Part model, mm, in its own coordinate system. Face numbers are marked on the shaded views. A direction names the side the tool comes from. Give positions to 0.01 mm unless a question says otherwise; leave off trailing zeros. Order: outer loops, then holes, each group sorted by start corner. A loop starts at its lowest first (then second) coordinate and runs counter-clockwise, first axis right, second up. Notation, with made-up numbers: (41, -6.5) -> (67, -6.5) arc R28 ccw to (67, 30.5) -> close; hole circle Ø6 at (23.5, -8.75). An arc over 180 degrees is marked (long way). Write item = value, one per line. Start each with the question number.
Item 1: Band-saw the part on D-D on x = 7. Write the cut outline in (y, z).
Item 2: Drill centre lines: line 1 along Y through (x, z) = (0, 2.8); line 2 along Y through (x, z) = (0, -15.7); line 3 along Z through (x, y) = (-9.25, 4.25). Where is each one in solid material? Low to high.
Item 3: Pull direction X, two halves, no side cores. Call the marked faces 3, 4 and 5: +X half, -X half, draft (parallel to the pull), parting line (faces both ways), or undercut.
Item 4: Band-saw the part on A-A on x = 0. Write the cut outline in (y, z).
Item 5: Tool access for the marked faces 1 and 2: list every direction of +Z, -Z, +X, -X, +Y, -Y with a clear straight run to the whole face (end or side of a thin tool).
Item 6: Band-saw the part on C-C on z = -10. Write the cut outline in (x, y), plus the area to 3 significant figures.
Item 7: Flat gauge pins, fed straight in: P1, Ø3, axis at x = -4.5, z = -7, coming from the -Y side; P2, Ø12, axis at x = -3.5, z = -11, coming from the -Y side; P3, Ø6, axis at x = 1, z = -8, coming from the +Y side. Where does each tip first touch, or does it go through?
Autodesk Inventor part; units mm, degrees
ref_plane "Work Plane1" through (0, 0, 0) normal (0, 0, 1) x (1, 0, 0)
ref_plane "Work Plane2" through (-23.495, -23.495, -13.97) normal (0, 0, -1) x (0, 1, 0)
ref_plane "YZ Plane" through (0, 0, 0) normal (1, 0, 0) x (0, 1, 0)
ref_plane "Work Plane1" through (0, 0, 0) normal (0, 0, 1) x (1, 0, 0)
sketch "Sketch1" plane through (0, 0, 0) normal (0, 0, 1) x (1, 0, 0)
  circle A0 centre (0, 0) radius 8.5725
  circle A1 centre (0, 0) radius 8.3185
  circle A2 centre (0, 0) radius 6.604
  point P0 (0, 0)
  dimension "d0" = 0.254
  dimension "d1" = 13.208
ref_plane "Work Plane2" through (-23.495, -23.495, -13.97) normal (0, 0, -1) x (0, 1, 0)
extrude "Extrusion1" add sketch "Sketch1" against normal up to surface (13.97 mm away) contours A1
sketch "Sketch2" plane through (0, 0, 0) normal (0, 0, 1) x (1, 0, 0)
  circle A0 centre (0, 0) radius 6.604
  circle A1 centre (0, 0) radius 8.3185
  circle A2 centre (0, 0) radius 10.8585
  dimension "d4" = 2.54
extrude "Extrusion2" add sketch "Sketch2" along normal blind 5.08 contours A1 | A2
sketch "Sketch4" plane through (0, 0, -13.97) normal (0, 0, -1) x (-1, 0, 0)
  circle A0 centre (0, 0) radius 6.604
  circle A1 centre (0, 0) radius 8.3185
  circle A2 centre (0, 0) radius 4.064
  dimension "d9" = 2.54
extrude "Extrusion4" add sketch "Sketch4" along normal blind 2.54 contours A0 | A1
properties part number "Big Bearing Sleeve"
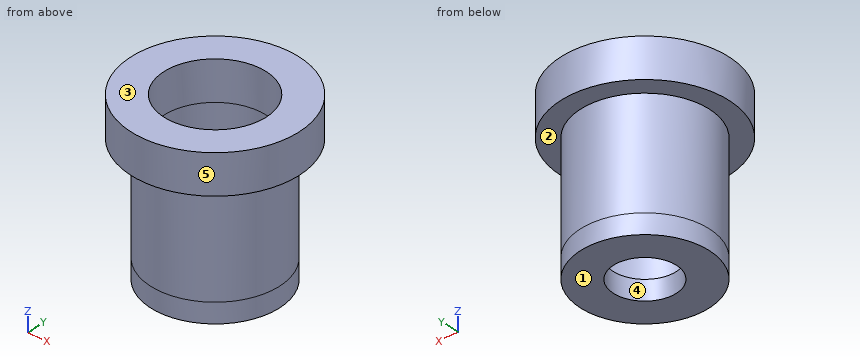
Values found:
q1.outline = (-8.3, 0) -> (-4.49, 0) -> (-4.49, -16.51) -> (4.49, -16.51) -> (4.49, 0) -> (8.3, 0) -> (8.3, 5.08) -> (-8.3, 5.08) -> close
q2.line_1 = -10.86 to -6.6, 6.6 to 10.86
q2.line_2 = -8.32 to -4.06, 4.06 to 8.32
q2.line_3 = 0 to 5.08
q3.face_3 = draft
q3.face_4 = undercut
q3.face_5 = parting line
q4.outline = (-10.86, 0) -> (-8.32, 0) -> (-8.32, -16.51) -> (-4.06, -16.51) -> (-4.06, -13.97) -> (-6.6, -13.97) -> (-6.6, 5.08) -> (-10.86, 5.08) -> close; (4.06, -16.51) -> (8.32, -16.51) -> (8.32, 0) -> (10.86, 0) -> (10.86, 5.08) -> (6.6, 5.08) -> (6.6, -13.97) -> (4.06, -13.97) -> close
q5.face_1 = -Z, +X, -X, +Y, -Y
q5.face_2 = -Z
q6.outline = circle Ø16.64 at (0, 0); hole circle Ø13.21 at (0, 0)
q6.area = 80.4 mm^2
q7.P1 = -7.76
q7.P2 = -8.32
q7.P3 = 8.32
